Geometry check sheet. Reference: the model listing, model coordinates, mm. A direction names the side the tool comes from. Give positions to 0.01 mm unless a question says otherwise; leave off trailing zeros. Write each loop counter-clockwise with the first axis right and the second up, starting at its lowest first coordinate (ties: lowest second). Pieces come first, ordered by that corner, then holes.
(1) Tool access check on faces 4 (the flat face through (56, 19, 12.7)), 5 (the flat face through (56, 75, 0)), 6 (the flat face through (56, 134, 12.7)). Record the directions out of +Z, -Z, +X, -X, +Y, -Y that give a thin tool (end or side, any length) a straight path to the whole face; none if there is none.
(2) Cross-section at C-C (y = 76.2). Record the boundary of the cut face in (x, z) (3 decimals), and give its area (3 significant figures).
(3) Cross-section at A-A (x = 23). Record the boundary of the cut face in (y, z) (3 decimals).
(4) Cross-section at B-B (z = 87). Record the boundary of the cut face in (x, y), and give its area (3 significant figures).
(5) Mould release check, pull along Y, two halves, no side actions. Record for faces 1 (the cylindrical face through (56.35, 76.898, 73.033)), 2 (the flat face through (56, 114.3, 58)), 3 (the flat face through (114.3, 75, 41)): +Y half, -Y half, draft (parallel to the pull), parting line (faces both ways), or undercut.
(6) Cross-section at D-D (z = 19.5). Record the boundary of the cut face in (x, y), and give its area (3 significant figures).
(7) Depth check by flat-ended pin: P1, Ø10, axis at x = 78, z = 53, coming from the +Y side; P2, Ø5, axis at x = 59, y = 45, coming from the -Z side; P3, Ø1.5, axis at y = 115.5, z = 43, coming from the -X side; P4, Ø4, axis at x = 96.5, y = 75, coming from the +Z side. Enter the tip coordinate at first touch or a pass-through.
(8) Thickness scan on line 1 along Z through (x, y) = (6.5, 20.5); line 2 along Y through (x, z) = (69, 38); line 3 along Y through (x, z) = (62.5, 89.5). Record the ranges inside material, lowest first.
```python
from build123d import *

# Parameters (mm, degrees)
F1_DEPTH = 114.3


with BuildPart() as f1:
    # F0 (on Right) → F1 (new body)
    with BuildSketch(Plane.YZ):
        with BuildLine():
            Line((0, 12.7), (0, 0))
            Line((0, 0), (152.4, 0))
            Line((152.4, 0), (152.4, 12.7))
            Line((152.4, 12.7), (114.3, 12.7))
            Line((114.3, 12.7), (114.3, 104.775))
            Line((114.3, 104.775), (107.95, 104.775))
            ThreePointArc((107.95, 104.775), (76.2, 73.025), (44.45, 104.775))
            Line((44.45, 104.775), (38.1, 104.775))
            Line((38.1, 104.775), (38.1, 12.7))
            Line((38.1, 12.7), (0, 12.7))
        make_face()
    extrude(amount=F1_DEPTH)


solid = f1.part
```
Reply:
1. face 4: +Z, +X, -X, -Y
1. face 5: -Z, +X, -X, +Y, -Y
1. face 6: +Z, +X, -X, +Y
2. outline: (0, 0) - (114.3, 0) - (114.3, 73.025) - (0, 73.025) - close
2. area: 8,350 mm2
3. outline: (0, 0) - (152.4, 0) - (152.4, 12.7) - (114.3, 12.7) - (114.3, 104.775) - (107.95, 104.775) arc R31.75 cw to (44.45, 104.775) - (38.1, 104.775) - (38.1, 12.7) - (0, 12.7) - close
4. outline: (0, 38.1) - (114.3, 38.1) - (114.3, 49.89) - (0, 49.89) - close; (0, 102.51) - (114.3, 102.51) - (114.3, 114.3) - (0, 114.3) - close
4. area: 2,700 mm2
5. face 1: undercut
5. face 2: +Y half
5. face 3: draft
6. outline: (0, 38.1) - (114.3, 38.1) - (114.3, 114.3) - (0, 114.3) - close
6. area: 8,710 mm2
7. P1: stops at y = 114.3
7. P2: stops at z = 0
7. P3: passes through
7. P4: stops at z = 73.19
8. line 1: z = 0 to 12.7
8. line 2: y = 38.1 to 114.3
8. line 3: y = 38.1 to 48.37, 104.03 to 114.3
